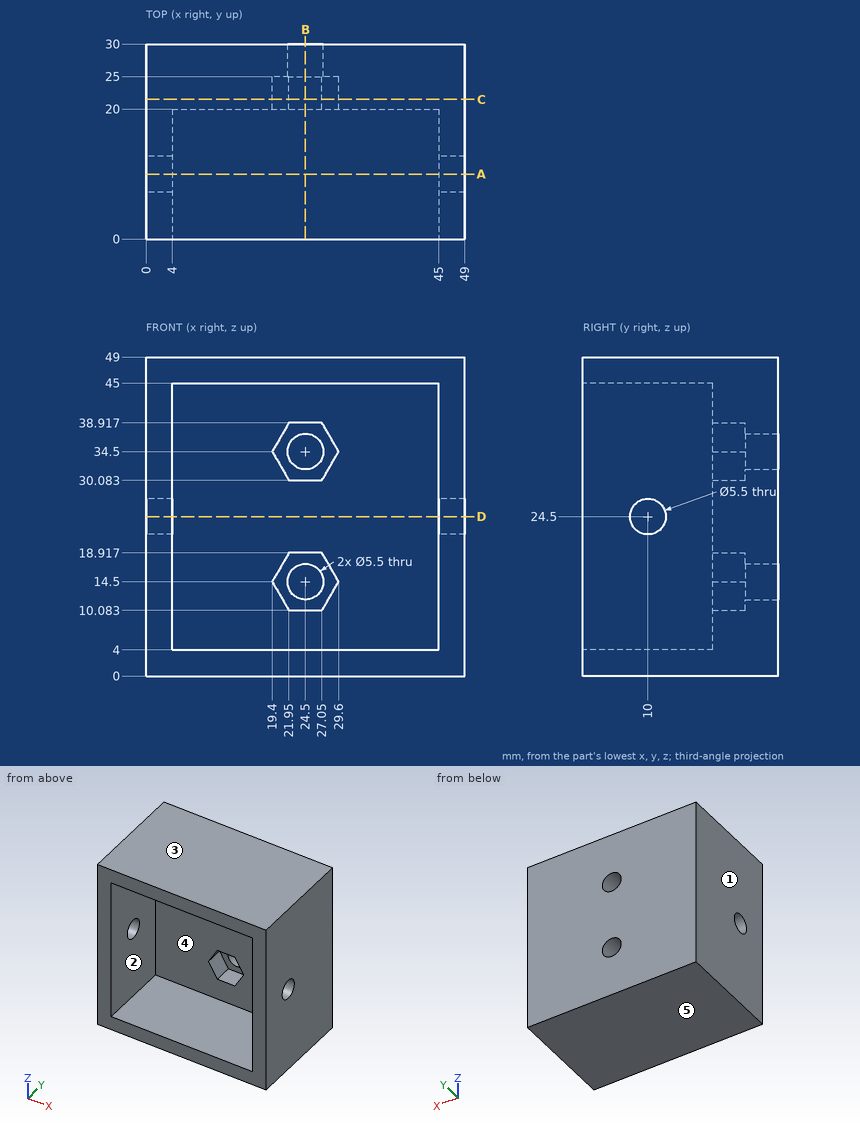
Here's the drawing with two shaded views (mm, measured from the low corner). I have some questions. A direction names the side the tool comes from. Round coordinates to 2 decimals unless told otherwise and drop trailing zeros. Write each loop counter-clockwise with the first axis right and the second up, starting at its lowest first coordinate (ties: lowest second). Pieces come first, ordered by that corner, then holes.
(1) Suppose I cut it at D-D on z = 24.5. Write out the boundary of the cut face in (x, y), and give its area (3 significant figures).
Findings below:
outline: (0, 0) - (4, 0) - (4, 7.25) - (0, 7.25) - close; (0, 12.75) - (4, 12.75) - (4, 20) - (45, 20) - (45, 12.75) - (49, 12.75) - (49, 30) - (0, 30) - close; (45, 0) - (49, 0) - (49, 7.25) - (45, 7.25) - close
area: 606 mm2
(2) If I drill on probe 1 along Z at (x, y) = (24.5, 26.4); probe 2 along X at (y, z) = (10.5, 30); probe 3 along Z at (x, y) = (46.05, 10), over which ranges is the centre line in solid material (lowest first)?
Findings below:
probe 1: z = 0 to 11.75, 17.25 to 31.75, 37.25 to 49
probe 2: x = 0 to 4, 45 to 49
probe 3: z = 0 to 21.75, 27.25 to 49
(3) Which directions (+Z, -Z, +X, -X, +Y, -Y) give clear straight access to the entire face, cutting with the end or side of a thin tool? Please do the marked faces 4 and 5.
Findings below:
face 4: -Y
face 5: -Z, +X, -X, +Y, -Y
(4) Thinking about a two-plate mould opening in X: for the marked faces 1, 2 and 3, which applies, +X half, -X half, draft (parallel to the pull), parting line (faces both ways), or undercut?
Findings below:
face 1: -X half
face 2: undercut
face 3: draft
(5) For pin 1 (4.5 mm diameter, centred on x = 23.5, z = 14.5, fed in from -Y); pin 2 (4.5 mm diameter, centred on y = 10, z = 24.5, fed in from +X), each with a flat end and sliding along its axis, tell me the tip position at first contact or that it passes through.
Findings below:
pin 1: stops at y = 25
pin 2: passes through
(6) Suppose I cut it at B-B on x = 24.5. Write out the boundary of the cut face in (y, z).
Findings below:
outline: (0, 0) - (30, 0) - (30, 11.75) - (25, 11.75) - (25, 10.08) - (20, 10.08) - (20, 4) - (0, 4) - close; (0, 45) - (20, 45) - (20, 38.92) - (25, 38.92) - (25, 37.25) - (30, 37.25) - (30, 49) - (0, 49) - close; (20, 18.92) - (25, 18.92) - (25, 17.25) - (30, 17.25) - (30, 31.75) - (25, 31.75) - (25, 30.08) - (20, 30.08) - close
(7) Suppose I cut it at C-C on y = 21.5. Write out the boundary of the cut face in (x, z), and give its area (3 significant figures).
Findings below:
outline: (0, 0) - (49, 0) - (49, 49) - (0, 49) - close; hole (19.4, 14.5) - (21.95, 10.08) - (27.05, 10.08) - (29.6, 14.5) - (27.05, 18.92) - (21.95, 18.92) - close; hole (19.4, 34.5) - (21.95, 30.08) - (27.05, 30.08) - (29.6, 34.5) - (27.05, 38.92) - (21.95, 38.92) - close
area: 2,270 mm2
(8) Suppose I cut it at A-A on y = 10. Write out the boundary of the cut face in (x, z), and give its area (3 significant figures).
Findings below:
outline: (0, 0) - (49, 0) - (49, 21.75) - (45, 21.75) - (45, 4) - (4, 4) - (4, 21.75) - (0, 21.75) - close; (0, 27.25) - (4, 27.25) - (4, 45) - (45, 45) - (45, 27.25) - (49, 27.25) - (49, 49) - (0, 49) - close
area: 676 mm2
